Verification items for this drawing (mm, ordinates from the low corner). A direction names the side the tool comes from. Coordinates: 2 decimals unless noted, no trailing zeros. Order: outer loops, then holes, each group sorted by start corner. A loop starts at its lowest first (then second) coordinate and runs counter-clockwise, first axis right, second up.
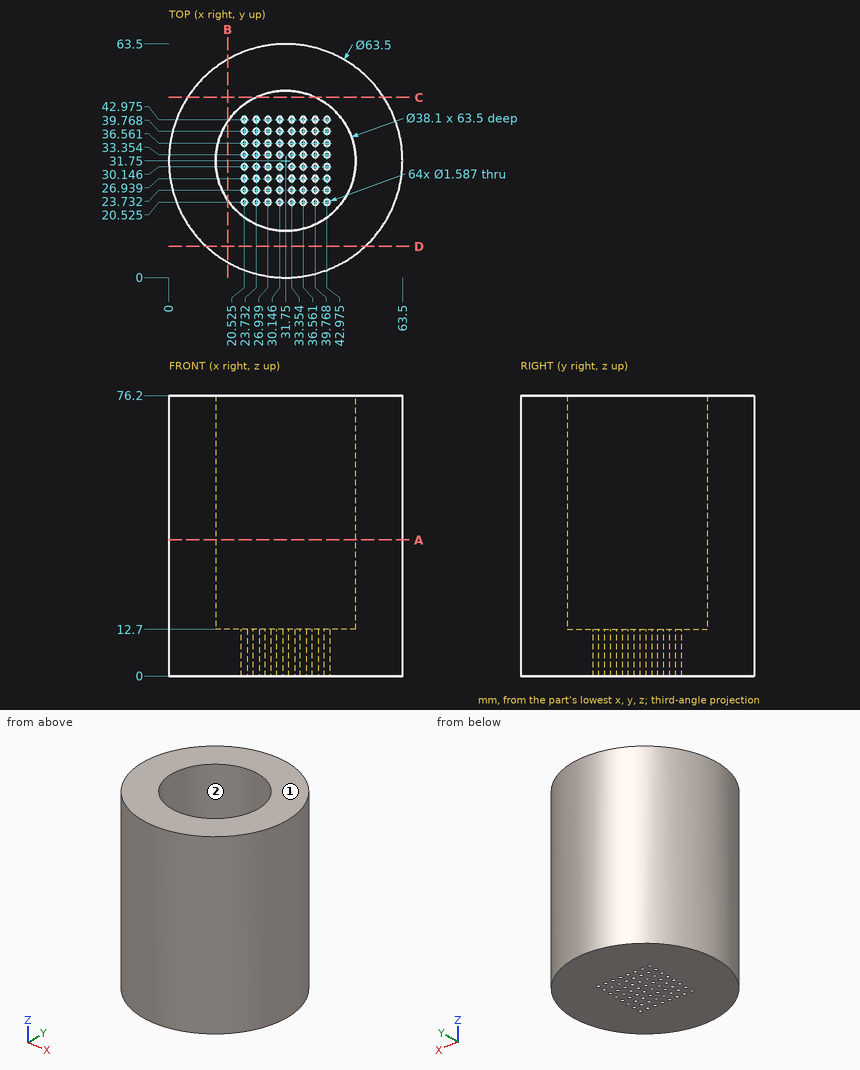
(1) Cross-section at C-C (y = 49). Enter the section's corners in (x, z) (1 decimal).
Filled in:
outline: (5.1, 0) - (58.4, 0) - (58.4, 76.2) - (39.8, 76.2) - (39.8, 12.7) - (23.7, 12.7) - (23.7, 76.2) - (5.1, 76.2) - close
(2) Cross-section at B-B (x = 16). Enter the section's corners in (y, z), and give its area (3 significant figures).
Filled in:
outline: (4.18, 0) - (59.32, 0) - (59.32, 76.2) - (42.47, 76.2) - (42.47, 12.7) - (21.03, 12.7) - (21.03, 76.2) - (4.18, 76.2) - close
area: 2,840 mm2
(3) Tool access check on the marked faces 1 and 2. Record the directions out of +Z, -Z, +X, -X, +Y, -Y that give a thin tool (end or side, any length) a straight path to the whole face; none if there is none.
Filled in:
face 1: +Z, +X, -X, +Y, -Y
face 2: +Z
(4) Cross-section at D-D (y = 8.5). Enter the section's corners in (x, z).
Filled in:
outline: (10.13, 0) - (53.37, 0) - (53.37, 76.2) - (10.13, 76.2) - close
(5) Go/stop test with flat-tipped pins: P1, Ø1.5, axis at x = 51.5, z = 63, coming from the -Y side; P2, Ø2.5, axis at x = 42.98, y = 36.56, coming from the -Z side; P3, Ø11.5, axis at x = 30.5, y = 30, coming from the +Z side; P4, Ø6, axis at y = 45.5, z = 45.5, coming from the -X side (1 decimal). Record where each tip stops, or that it passes through.
Filled in:
P1: stops at y = 6.31
P2: stops at z = 0
P3: stops at z = 12.7
P4: stops at x = 1.9
(6) Thickness scan on probe 1 along Z at (x, y) = (41, 44.5); probe 2 along Y at (x, z) = (28, 43); probe 3 along Y at (x, z) = (36.5, 25.5). Record the ranges inside material, lowest first.
Filled in:
probe 1: z = 0 to 12.7
probe 2: y = 0.22 to 13.07, 50.43 to 63.28
probe 3: y = 0.36 to 13.3, 50.2 to 63.14
(7) Cross-section at A-A (z = 37). Enter the section's corners in (x, y).
Filled in:
outline: circle Ø63.5 at (31.75, 31.75); hole circle Ø38.1 at (31.75, 31.75)
